The model under review builds one solid part; all positions refer to its coordinate system, in mm. A direction names the side the tool comes from. Give positions to 0.01 mm unless a question says otherwise; leave off trailing zeros. Write each loop counter-clockwise with the first axis right and the second up, starting at its lowest first coordinate (ties: lowest second). Pieces come first, ordered by that corner, then holes. Notation, with made-up numbers: M 6,81 L 26,81 A11 cw 26,92 Z; hole C 24,77.25 d4. An arc over 180 degrees is marked long. Write each question's results on one line, items separated by ' | '. Start each with the question number.
from build123d import *

# Parameters (mm, degrees)
F1_DEPTH = 50.8
F3_DEPTH = 25.4
F5_DEPTH = 66.549
F6_R     = 3.9624
F7_DEPTH = 12.701
F6_R_2   = 6.35
F8_DEPTH = 6.096


with BuildPart() as f1:
    # F0 (on Front) → F1 (new body)
    with BuildSketch(Plane.XZ):
        Polygon((0, 12.7), (0, 0), (85.852, 0), (131.70327, -45.85127), (149.663782, -27.890758), (111.587496, 10.185528), (102.60724, 1.205272), (91.112512, 12.7), align=None)
    extrude(amount=F1_DEPTH)

    # F2 (on face) → F3 (cut)
    with BuildSketch(Plane(origin=(60.886512, 0, 60.886512), x_dir=(0.707107, 0, -0.707107), z_dir=(0.707107, 0, 0.707107))):
        with BuildLine():
            Line((125.550019, -50.8), (125.550019, -25.4))
            ThreePointArc((125.550019, -25.4), (123.934026, -38.492922), (119.183037, -50.8))
            Line((119.183037, -50.8), (125.550019, -50.8))
        make_face()
        with BuildLine():
            Line((125.550019, -25.4), (125.550019, 0))
            Line((125.550019, 0), (119.183037, 0))
            ThreePointArc((119.183037, 0), (123.934026, -12.307078), (125.550019, -25.4))
        make_face()
    extrude(amount=-F3_DEPTH, mode=Mode.SUBTRACT)

    # F4 (on face) → F5 (cut, through all)
    with BuildSketch(Plane(origin=(50.700984, 0, -50.700984), x_dir=(0, -1, 0), z_dir=(-0.707107, 0, 0.707107))):
        Polygon((41.148, 80.010531), (35.052, 80.010531), (35.052, 86.106531), (15.748, 86.106531), (15.748, 80.010531), (9.652, 80.010531), (9.652, 73.406531), (41.148, 73.406531), align=None)
    extrude(amount=-F5_DEPTH, mode=Mode.SUBTRACT)

    # F6 (on face) → F7 (cut, through all)
    with BuildSketch(Plane(origin=(0, 0, 0), x_dir=(1, 0, 0), z_dir=(0, 0, -1))):
        with Locations((15.748, 12.7)):
            Circle(F6_R)
        with Locations((15.748, 38.1)):
            Circle(F6_R)
        with Locations((69.596, 38.1)):
            Circle(F6_R)
        with Locations((69.596, 12.7)):
            Circle(F6_R)
    extrude(amount=-F7_DEPTH, mode=Mode.SUBTRACT)

    # F6 (on face) → F8 (cut)
    with BuildSketch(Plane(origin=(0, 0, 0), x_dir=(1, 0, 0), z_dir=(0, 0, -1))):
        with Locations((15.748, 12.7)):
            Circle(F6_R_2)
        with Locations((15.748, 12.7)):
            Circle(F6_R, mode=Mode.SUBTRACT)
        with Locations((15.748, 38.1)):
            Circle(F6_R_2)
        with Locations((15.748, 38.1)):
            Circle(F6_R, mode=Mode.SUBTRACT)
        with Locations((69.596, 12.7)):
            Circle(F6_R_2)
        with Locations((69.596, 12.7)):
            Circle(F6_R, mode=Mode.SUBTRACT)
        with Locations((69.596, 38.1)):
            Circle(F6_R_2)
        with Locations((69.596, 38.1)):
            Circle(F6_R, mode=Mode.SUBTRACT)
    extrude(amount=-F8_DEPTH, mode=Mode.SUBTRACT)


solid = f1.part
(1) Add section D-D (x = 115). State the section outline as (y, z) points, then the cut area to 3 significant figures.
(2) Draft analysis for pull direction X (two halves, no side actions). For faces 6 (the flat face through (88.4, -50.8, -2.2)), 7 (the flat face through (0, -25, 6)), 8 (the flat face through (74, -38, 6.096)), state which applies: pulls with the +X half, pulls with the -X half, needs draft (parallel to the pull), parting line crosses it, or undercut.
(3) Clearance check with flat-ended pins moving along their axes: P1, Ø4, axis at x = 72.5, y = -40, coming from the -Z side; P2, Ø1.5, axis at x = 101, y = -40.5, coming from the +Z side; P3, Ø5, axis at y = -40.5, z = -30, coming from the +X side. State where each tip first meets the part, or that it passes through.
(4) Wall thickness on L1, parallel to Y at x = 70, z = 8; L2, parallel to Y at x = 113.5, z = 8; L3, parallel to Y at x = 13.5, z = 5.5: over which ranges is each line inside the solid? List them lowest first.
(5) Add section C-C (y = -3.5). State the section outline as (x, z) points, then the cut area to 3 significant figures.
(6) Add section A-A (x = 16.5). State the section outline as (y, z) points, then the cut area to 3 significant figures.
(7) Add section B-B (y = -39.5). State the section outline as (x, z) points (1 decimal), then the cut area to 3 significant figures.
(8) Machinability: for faces 1 (the cylindrical face through (73.01, -18.054, 3.005)), 2 (the flat face through (108.2, -44.6, 6.8)), 3 (the flat face through (125.74, -12.74, -12.59)), 4 (the flat face through (128, -35.052, -10)), 5 (the flat face through (42, -25, 0)), which of the approach directions +Z, -Z, +X, -X, +Y, -Y give a long, thin tool a straight path to every point of the face, cutting with its end or side? Answer none if there is none.
Calculated:
1) outline: M -50.8,-29.15 L 0,-29.15 L 0,6.77 L -15.75,6.77 L -15.75,-1.85 L -9.65,-1.85 L -9.65,-11.19 L -41.15,-11.19 L -41.15,-1.85 L -35.05,-1.85 L -35.05,6.77 L -50.8,6.77 Z | area: 1,360 mm²
2) face 6: needs draft | face 7: pulls with the -X half | face 8: undercut
3) P1: stops at z = 6.1 | P2: stops at z = 3.56 | P3: stops at x = 147.19
4) L1: y = -50.8 to -42.04, -34.16 to -16.64, -8.76 to 0 | L2: y = -50.8 to -35.05, -15.75 to 0 | L3: y = -50.8 to -44.04, -32.16 to -18.64, -6.76 to 0
5) outline: M 0,0 L 85.85,0 L 128.41,-42.56 L 146.37,-24.6 L 111.59,10.19 L 102.61,1.21 L 91.11,12.7 L 0,12.7 Z | area: 2,550 mm²
6) outline: M -50.8,0 L -44.41,0 L -44.41,6.1 L -41.99,6.1 L -41.99,12.7 L -50.8,12.7 Z; M -34.21,6.1 L -31.79,6.1 L -31.79,0 L -19.01,0 L -19.01,6.1 L -16.59,6.1 L -16.59,12.7 L -34.21,12.7 Z; M -8.81,6.1 L -6.39,6.1 L -6.39,0 L 0,0 L 0,12.7 L -8.81,12.7 Z | area: 389 mm²
7) outline: M 0,0 L 9.6,0 L 9.6,6.1 L 12,6.1 L 12,12.7 L 0,12.7 Z; M 19.5,6.1 L 21.9,6.1 L 21.9,0 L 63.4,0 L 63.4,6.1 L 65.9,6.1 L 65.9,12.7 L 19.5,12.7 Z; M 73.3,6.1 L 75.8,6.1 L 75.8,0 L 85.9,0 L 130.4,-44.5 L 139.4,-35.5 L 91.1,12.7 L 73.3,12.7 Z; M 107.3,5.9 L 144,-30.9 L 148.3,-26.6 L 111.6,10.2 Z | area: 2,020 mm²
8) face 1: -Z | face 2: +Z, +Y, -Y | face 3: none | face 4: +Z, +X | face 5: -Z, -X, +Y, -Y
